from build123d import *

# Parameters (mm, degrees)
SKETCH_R           = 3
SKETCH_R_2         = 6.15
PAD_DEPTH          = 15
FILLET_R           = 5
SKETCH001_R        = 2.45
POCKET_DEPTH       = 11
POLARPATTERN_COUNT = 3


with BuildPart() as part:
    # Sketch → Pad (new body)
    with BuildSketch(Plane.XY):
        Polygon((0, 23.5333333333), (-20.3804645024, -11.7666666667), (20.3804645024, -11.7666666667), align=None)
        with Locations((0, 13.7)):
            Circle(SKETCH_R, mode=Mode.SUBTRACT)
        with Locations((11.8645480319, -6.85)):
            Circle(SKETCH_R, mode=Mode.SUBTRACT)
        with Locations((-11.8645480318, -6.85)):
            Circle(SKETCH_R, mode=Mode.SUBTRACT)
        Circle(SKETCH_R_2, mode=Mode.SUBTRACT)
    extrude(amount=PAD_DEPTH)

    # Fillet
    fillet_edges = [part.edges().sort_by_distance(p)[0] for p in [
        (-20.380465, -11.766667, 7.5),
        (0, 23.533333, 7.5),
        (20.380465, -11.766667, 7.5),
    ]]
    fillet(fillet_edges, radius=FILLET_R)

    # Sketch001 (on DatumPlane) → Pocket (cut)
    with BuildSketch(Plane(origin=(-10.1902322512, 5.8833333333, 0), x_dir=(-0.5, -0.8660254038, 0), z_dir=(-0.8660254038, 0.5, 0))):
        with Locations((0, 7.5)):
            Circle(SKETCH001_R)
    pocket = extrude(amount=-POCKET_DEPTH, mode=Mode.SUBTRACT)

    # PolarPattern: Pocket ×3 about axis
    polarpattern_axis = Axis((0, 0, 0), (0, 0, 1))
    for i in range(1, POLARPATTERN_COUNT):
        add(pocket.rotate(polarpattern_axis, i * 360 / POLARPATTERN_COUNT), mode=Mode.SUBTRACT)


solid = part.part
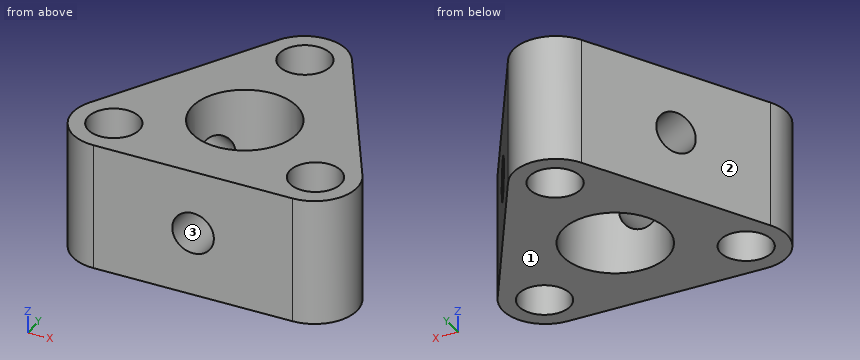
Input: part model. Units: mm. Frame: model coordinates. Face numbers are marked on the shaded views. Give positions to 0.01 mm unless a question says otherwise; leave off trailing zeros. Order: outer loops, then holes, each group sorted by start corner. A loop starts at its lowest first (then second) coordinate and runs counter-clockwise, first axis right, second up. Notation, with made-up numbers: (-5, -23.5) - (39, -23.5) arc R20 cw to (39, 0.5) - close; hole circle Ø10 at (-15, 87.25). An arc over 180 degrees is marked (long way). Answer as a JSON object with one key per item and string values. Group by question number.
Q1. Cut plane D-D, the plane z = 7.5. Output: boundary loops of the cut face in (x, y), then the cut area to 3 significant figures.
Q2. Cut plane B-B, the plane y = -6.85. Output: boundary loops of the cut face in (x, z), then the cut area to 3 significant figures.
Q3. Cut plane C-C, the plane z = 3.25. Output: boundary loops of the cut face in (x, y), then the cut area to 3 significant figures.
Q4. First-contact query: pin 1 Ø7 at (x, y) = (0, 13.7) entering from -Z; pin 2 Ø6 at (y, z) = (10.5, 5) entering from -X; pin 3 Ø1.5 at (x, z) = (5, 8) entering from +Y; pin 4 Ø1 at (y, z) = (-0.5, 6.5) entering from +X. Flat tips, straight axial feed; report the tip coordinate or a pass-through.
Q5. Line query: probe 1 along X at (y, z) = (-8, 8.5); probe 2 along Z at (x, y) = (0, -8.25); probe 3 along Y at (x, z) = (-2.5, 12.25). Output: solid intervals per line, ascending.
Q6. Mould query, pull axis X, two halves, no side actions, for the marked faces 1, 2 and 3. Classes: pulls with the +X half, pulls with the -X half, needs draft (parallel to the pull), parting line crosses it, or undercut.
Q7. Cut plane A-A, the plane x = 0. Output: boundary loops of the cut face in (y, z), then the cut area to 3 significant figures.
Results:
{
 "1": {"outline": "(-16.05, -4.27) arc R5 ccw to (-11.72, -11.77) - (-2.45, -11.77) - (-2.45, -5.64) arc R6.15 cw to (-6.11, 0.7) - (-11.42, 3.76) - close; (-8.97, 8.01) - (-3.66, 4.94) arc R6.15 cw to (3.66, 4.94) - (8.97, 8.01) - (4.33, 16.03) arc R5 ccw to (-4.33, 16.03) - close; (2.45, -11.77) - (11.72, -11.77) arc R5 ccw to (16.05, -4.27) - (11.42, 3.76) - (6.11, 0.7) arc R6.15 cw to (2.45, -5.64) - close; hole circle Ø6 at (-11.86, -6.85); hole circle Ø6 at (0, 13.7); hole circle Ø6 at (11.86, -6.85)", "area": "379 mm^2"},
 "2": {"outline": "(-16.72, 0) - (-14.86, 0) - (-14.86, 15) - (-16.72, 15) - close; (-8.86, 0) - (8.86, 0) - (8.86, 15) - (-8.86, 15) - close; (14.86, 0) - (16.72, 0) - (16.72, 15) - (14.86, 15) - close; hole circle Ø4.9 at (0, 7.5)", "area": "303 mm^2"},
 "3": {"outline": "(-16.05, -4.27) arc R5 ccw to (-11.72, -11.77) - (11.72, -11.77) arc R5 ccw to (16.05, -4.27) - (4.33, 16.03) arc R5 ccw to (-4.33, 16.03) - close; hole circle Ø6 at (-11.86, -6.85); hole circle Ø12.3 at (0, 0); hole circle Ø6 at (0, 13.7); hole circle Ø6 at (11.86, -6.85)", "area": "464 mm^2"},
 "4": {"pin 1": "z = 0", "pin 2": "x = -9.26", "pin 3": "y = 16.17", "pin 4": "x = 14.16"},
 "5": {"probe 1": "-16.57 to -14.64, -9.09 to -2.24, 2.24 to 9.09, 14.64 to 16.57", "probe 2": "0 to 5.05, 9.95 to 15", "probe 3": "-11.77 to -5.62, 5.62 to 12.04, 15.36 to 17.86"},
 "6": {"face 1": "needs draft", "face 2": "pulls with the -X half", "face 3": "undercut"},
 "7": {"outline": "(-11.77, 0) - (-6.15, 0) - (-6.15, 5.05) - (-11.77, 5.05) - close; (-11.77, 9.95) - (-6.15, 9.95) - (-6.15, 15) - (-11.77, 15) - close; (6.15, 0) - (10.7, 0) - (10.7, 15) - (6.15, 15) - close; (16.7, 0) - (18.53, 0) - (18.53, 15) - (16.7, 15) - close", "area": "152 mm^2"}
}
